Part model, mm, in its own coordinate system. A direction names the side the tool comes from. Round coordinates to 2 decimals unless told otherwise and drop trailing zeros. Loops run counter-clockwise (first coordinate to the right, second up) from the corner with the lowest first, then second, coordinate; pieces in that order, holes last.
1) Band-saw the part on C-C, the plane z = 24.5. Write the cut outline in (x, y), then the cut area to 3 significant figures.
2) Mould opens along Z. For faces 6 (the cylindrical face through (1.707, -1.503, 66.177)), 7 (the cylindrical face through (-6.81, -1.5, -6.66)), 8 (the flat face through (12.68, -1.5, 89.56)), 9 (the cylindrical face through (-0.69, -1.5, -3.1)) say: +Z half, -Z half, draft (parallel to the pull), parting line (faces both ways), or undercut.
3) Band-saw the part on A-A, the plane x = 14. Write the cut outline in (y, z).
4) Drop flat-ended pins along their axis: P1, Ø5, axis at x = 0, z = 0, coming from the +Y side; P2, Ø1.5, axis at y = -2.5, z = 16.5, coming from the -X side. Give the stop position or say it passes through.
5) Band-saw the part on B-B, the plane y = -0.55. State how many separate pieces and enclosed holes the cut face has, then the cut area to 3 significant figures.
6) Probe line 1 (X direction, y = -0.7, z = 101.5); line 2 (X direction, y = -1.9, z = 117); line 3 (Z direction, x = -4, y = -1.15). List the from-to ranges inside material, lowest first.
7) 3-axis set-ups, long thin cutter, end or side, ignore diameter. For faces 1 (the flat face through (13.412, -1.503, 38.384)), 2 (the flat face through (3, 0, 43)), 3 (the flat face through (3, -3.048, 43)), 4 (the cylindrical face through (13.3, -1.5, 9.18)), 5 (the flat face through (31.9, -1.5, 7.36)): which of +Z, -Z, +X, -X, +Y, -Y reach the whole face in a straight line?
8) Band-saw the part on D-D, the plane x = 26. Write the cut outline in (y, z), then the cut area to 3 significant figures.
from build123d import *

# Parameters (mm, degrees)
F0_R     = 3.175
F0_R_2   = 2.935696
F1_DEPTH = 3.048


with BuildPart() as f1:
    # F0 (on Front) → F1 (new body)
    with BuildSketch(Plane.XZ):
        with BuildLine():
            ThreePointArc((0.677344, -9.500886), (6.970557, -6.491299), (9.525, 0))
            ThreePointArc((9.525, 0), (0, 9.525), (-9.525, 0))
            ThreePointArc((-9.525, 0), (-6.735192, -6.735192), (0, -9.525))
            Line((0, -9.525), (0.677344, -9.500886))
        make_face()
        Circle(F0_R, mode=Mode.SUBTRACT)
        with BuildLine():
            ThreePointArc((-9.525, 0), (0, 9.525), (9.525, 0))
            ThreePointArc((9.525, 0), (6.970557, -6.491299), (0.677344, -9.500886))
            Line((0.677344, -9.500886), (44.732405, -7.932475))
            ThreePointArc((44.732405, -7.932475), (36.519221, -0.326571), (44.079274, 7.928838))
            Line((44.079274, 7.928838), (19.377548, 6.773866))
            ThreePointArc((19.377548, 6.773866), (13.234292, 9.248177), (11.096492, 15.51648))
            Line((11.096492, 15.51648), (15.794203, 61.90038))
            ThreePointArc((15.794203, 61.90038), (0, 47.625), (-15.794203, 61.90038))
            Line((-15.794203, 61.90038), (-9.525, 0))
        make_face()
        with BuildLine():
            ThreePointArc((0, -9.525), (0.338886, -9.51897), (0.677344, -9.500886))
            Line((0.677344, -9.500886), (0, -9.525))
        make_face()
        with BuildLine():
            ThreePointArc((-15.747457, 65.508289), (-15.873668, 63.705667), (-15.794203, 61.90038))
            ThreePointArc((-15.794203, 61.90038), (0, 47.625), (15.794203, 61.90038))
            ThreePointArc((15.794203, 61.90038), (15.854788, 62.699171), (15.875, 63.5))
            ThreePointArc((15.875, 63.5), (15.843082, 64.506168), (15.747457, 65.508289))
            ThreePointArc((15.747457, 65.508289), (0, 79.375), (-15.747457, 65.508289))
        make_face()
        with Locations((0, 63.5)):
            Circle(F0_R, mode=Mode.SUBTRACT)
        with BuildLine():
            ThreePointArc((44.079274, 7.928838), (36.519221, -0.326571), (44.732405, -7.932475))
            ThreePointArc((44.732405, -7.932475), (50.161633, -5.51191), (52.3875, 0))
            ThreePointArc((52.3875, 0), (49.930021, 5.742236), (44.079274, 7.928838))
        make_face()
        with Locations((44.45, 0)):
            Circle(F0_R, mode=Mode.SUBTRACT)
        with BuildLine():
            Line((-9.525, 114.3), (-15.747457, 65.508289))
            ThreePointArc((-15.747457, 65.508289), (0, 79.375), (15.747457, 65.508289))
            Line((15.747457, 65.508289), (9.525, 114.3))
            ThreePointArc((9.525, 114.3), (0, 104.775), (-9.525, 114.3))
        make_face()
        with Locations((-3.175, 100.0252)):
            Circle(F0_R_2, mode=Mode.SUBTRACT)
        with BuildLine():
            ThreePointArc((9.525, 114.3), (0, 123.825), (-9.525, 114.3))
            ThreePointArc((-9.525, 114.3), (0, 104.775), (9.525, 114.3))
        make_face()
        with Locations((0, 114.3)):
            Circle(F0_R, mode=Mode.SUBTRACT)
    extrude(amount=F1_DEPTH)


solid = f1.part
Reported:
1. outline: (-12.01, -3.05) - (12.01, -3.05) - (12.01, 0) - (-12.01, 0) - close
1. area: 73.2 mm2
2. face 6: undercut
2. face 7: -Z half
2. face 8: +Z half
2. face 9: undercut
3. outline: (-3.05, -9.03) - (0, -9.03) - (0, 8.54) - (-3.05, 8.54) - close; (-3.05, 44.18) - (0, 44.18) - (0, 79.21) - (-3.05, 79.21) - close
4. P1: passes through
4. P2: stops at x = -11.27
5. separate pieces: 1
5. enclosed holes: 5
5. area: 3,730 mm2
6. line 1: x = -11.16 to -5.71, -0.64 to 11.16
6. line 2: x = -9.13 to -1.67, 1.67 to 9.13
6. line 3: z = -8.64 to 97.21, 102.84 to 122.94
7. face 1: +X, +Y, -Y
7. face 2: +Z, -Z, +X, -X, +Y
7. face 3: +Z, -Z, +X, -X, -Y
7. face 4: +Y, -Y
7. face 5: +Z, +Y, -Y
8. outline: (-3.05, -8.6) - (0, -8.6) - (0, 7.08) - (-3.05, 7.08) - close
8. area: 47.8 mm2
